Source: three-view drawing plus pictorial views. Frame: mm from the lowest corner of the part. A direction names the side the tool comes from. Give positions to 0.01 mm unless a question says otherwise; leave off trailing zeros. Loops run counter-clockwise (first coordinate to the right, second up) from the corner with the lowest first, then second, coordinate; pieces in that order, holes last.
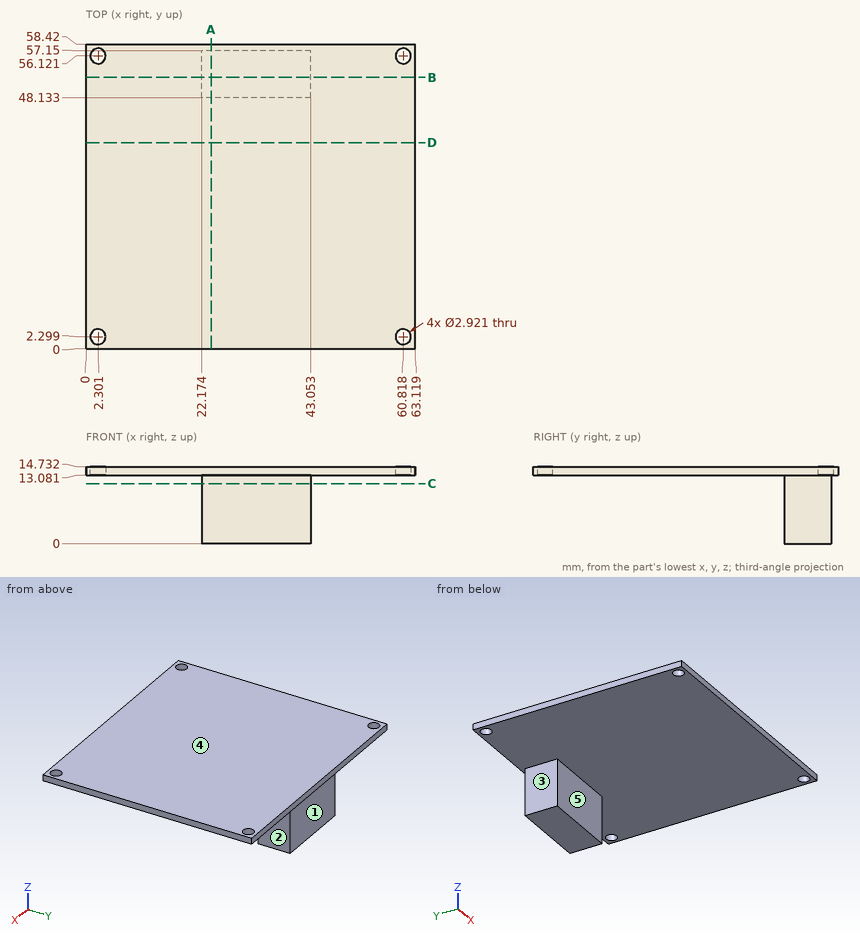
(1) Cut plane B-B (y = 52). Return the cut outline in (x, z), and give its area (3 significant figures).
Values follow:
outline: (0, 13.08) - (22.17, 13.08) - (22.17, 0) - (43.05, 0) - (43.05, 13.08) - (63.12, 13.08) - (63.12, 14.73) - (0, 14.73) - close
area: 377 mm2
(2) Pin query (flat end, axial travel): pin 1 Ø7 at (y, z) = (51, 8) entering from +X; pin 2 Ø4.5 at (y, z) = (54.5, 7) entering from -X; pin 3 Ø1.5 at (x, z) = (33.5, 8.5) entering from -Y; pin 4 Ø2.5 at (x, y) = (60.82, 2.3) entering from -Z. Return the tip coordinate at first contact, or that it passes through.
Values follow:
pin 1: stops at x = 43.05
pin 2: stops at x = 22.17
pin 3: stops at y = 48.13
pin 4: passes through
(3) Cut plane C-C (z = 11.5). Return the cut outline in (x, y), and give its area (3 significant figures).
Values follow:
outline: (22.17, 48.13) - (43.05, 48.13) - (43.05, 57.15) - (22.17, 57.15) - close
area: 188 mm2
(4) Cut plane D-D (y = 39.5). Return the cut outline in (x, z).
Values follow:
outline: (0, 13.08) - (63.12, 13.08) - (63.12, 14.73) - (0, 14.73) - close
(5) Reachability of the marked faces 1, 2, 3, 4 and 5 from +Z, -Z, +X, -X, +Y, -Y: full face, straight path, thin tool, end or side. Return the list, or none.
Values follow:
face 1: -Z, +X, -X, +Y
face 2: -Z, +X, +Y, -Y
face 3: -Z, -X, +Y, -Y
face 4: +Z, +X, -X, +Y, -Y
face 5: -Z, +X, -X, -Y
(6) Cut plane A-A (x = 24). Return the cut outline in (y, z), and give its area (3 significant figures).
Values follow:
outline: (0, 13.08) - (48.13, 13.08) - (48.13, 0) - (57.15, 0) - (57.15, 13.08) - (58.42, 13.08) - (58.42, 14.73) - (0, 14.73) - close
area: 214 mm2
(7) Ray query, probe 1 along Z at (x, y) = (24, 33); probe 2 along X at (y, z) = (51, 4.25); probe 3 along Y at (x, z) = (38, 9). Return the intervals inside material, ascending.
Values follow:
probe 1: z = 13.08 to 14.73
probe 2: x = 22.17 to 43.05
probe 3: y = 48.13 to 57.15
